```python
from build123d import *


with BuildPart() as part:
    # Esquisse1 → Révolution1 (revolve)
    with BuildSketch(Plane.XY, mode=Mode.PRIVATE) as r_volution1_sk:
        Polygon((0, 0), (27.5, 0), (27.5, 3), (24.5, 3), (24.5, 5), (17.5, 12), (15.5, 12), (15.5, 14), (8, 14), (8, 17), (6, 17), (6, 92), (0, 92), align=None)
    revolve(r_volution1_sk.sketch.rotate(Axis((0, 92, 0), (0, -1, 0)), 90), axis=Axis((0, 92, 0), (0, -1, 0)))


solid = part.part
```
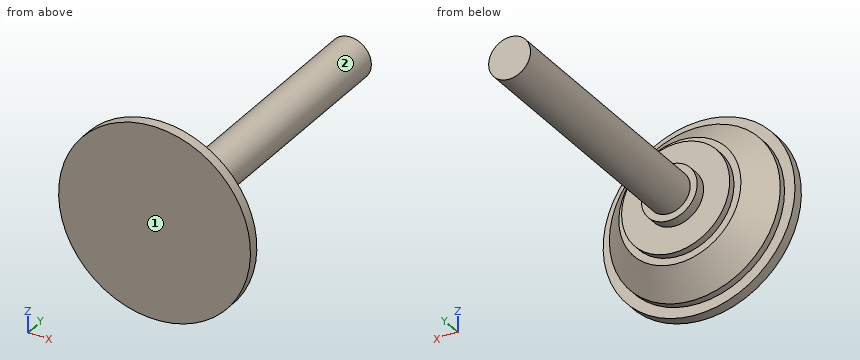
Check sheet for the modelled part. Datum: model origin and axes. Units: mm. Face numbers are marked on the shaded views. A direction names the side the tool comes from. Round coordinates to 2 decimals unless told otherwise and drop trailing zeros. Order: outer loops, then holes, each group sorted by start corner. A loop starts at its lowest first (then second) coordinate and runs counter-clockwise, first axis right, second up. Notation, with made-up numbers: (25.25, 88) - (38.25, 88) arc R15 ccw to (38.25, 108) - close; hole circle Ø6 at (-10, 0). An arc over 180 degrees is marked (long way). Write item = value, one per line.
Q1. Section check D-D (y = 9). Record the boundary of the cut face in (x, z).
Computed:
outline = circle Ø41 at (0, 0)
Q2. Go/stop test with flat-tipped pins: pin 1 (12 mm diameter, centred on x = 16, y = 61, fed in from -Z); pin 2 (12 mm diameter, centred on x = -11.5, y = 61, fed in from +Z); pin 3 (12 mm diameter, centred on x = 0, y = 75, fed in from +Z); pin 4 (8 mm diameter, centred on y = 11, z = -18.5, fed in from -X). Record where each tip stops, or that it passes through.
Computed:
pin_1 = through
pin_2 = 2.4
pin_3 = 6
pin_4 = -14.55
Q3. Section check B-B (z = 0). Record the boundary of the cut face in (x, y).
Computed:
outline = (-27.5, 0) - (27.5, 0) - (27.5, 3) - (24.5, 3) - (24.5, 5) - (17.5, 12) - (15.5, 12) - (15.5, 14) - (8, 14) - (8, 17) - (6, 17) - (6, 92) - (-6, 92) - (-6, 17) - (-8, 17) - (-8, 14) - (-15.5, 14) - (-15.5, 12) - (-17.5, 12) - (-24.5, 5) - (-24.5, 3) - (-27.5, 3) - close
Q4. Section check A-A (x = 0). Record the boundary of the cut face in (y, z), and give its area (3 significant figures).
Computed:
outline = (0, -27.5) - (3, -27.5) - (3, -24.5) - (5, -24.5) - (12, -17.5) - (12, -15.5) - (14, -15.5) - (14, -8) - (17, -8) - (17, -6) - (92, -6) - (92, 6) - (17, 6) - (17, 8) - (14, 8) - (14, 15.5) - (12, 15.5) - (12, 17.5) - (5, 24.5) - (3, 24.5) - (3, 27.5) - (0, 27.5) - close
area = 1,570 mm^2
Q5. Section check C-C (y = 20.5). Record the boundary of the cut face in (x, z), and give its area (3 significant figures).
Computed:
outline = circle Ø12 at (0, 0)
area = 113 mm^2
Q6. Thickness scan on line 1 along Y through (x, z) = (9, 6); line 2 along Y through (x, z) = (-11, 19.5); line 3 along X through (y, z) = (5.5, -13). Record the ranges inside material, lowest first.
Computed:
line_1 = 0 to 14
line_2 = 0 to 7.11
line_3 = -20.17 to 20.17
Q7. Tool access check on the marked faces 1 and 2. Record the directions out of +Z, -Z, +X, -X, +Y, -Y that give a thin tool (end or side, any length) a straight path to the whole face; none if there is none.
Computed:
face_1 = +Z, -Z, +X, -X, -Y
face_2 = +Y
